Check sheet for the drawn part. Datum: minimum x, y, z corner. Units: mm. Coordinates: 2 decimals unless noted, no trailing zeros. Loops run counter-clockwise (first coordinate to the right, second up) from the corner with the lowest first, then second, coordinate; pieces in that order, holes last.
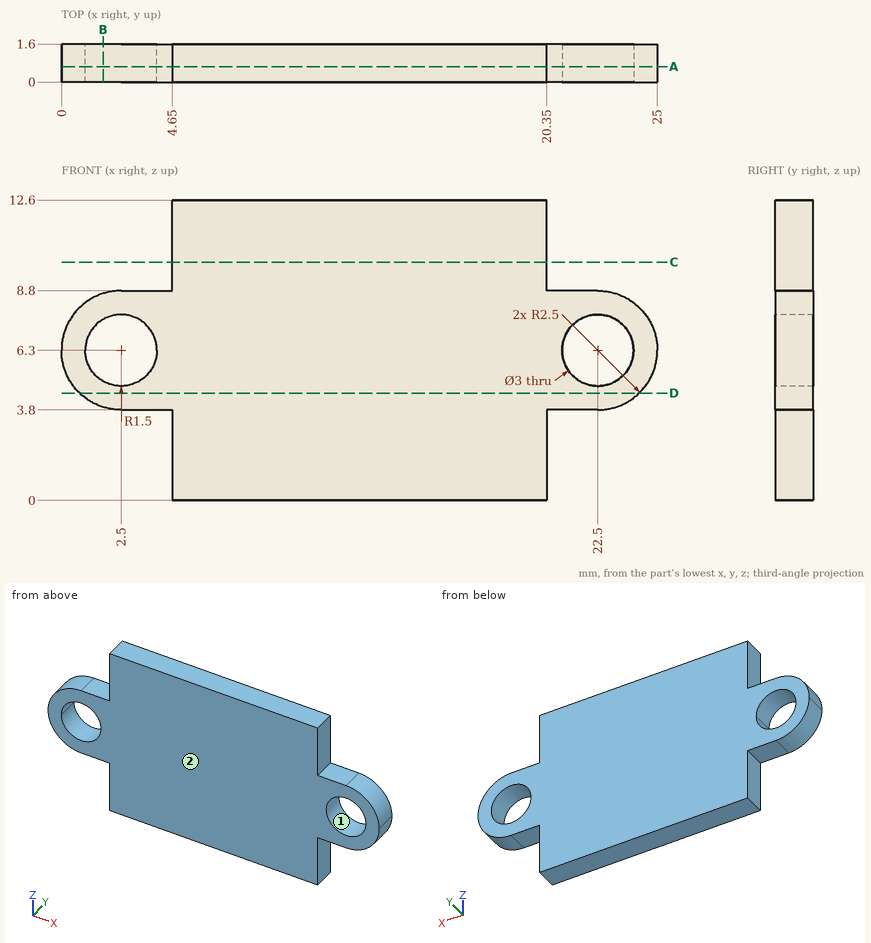
1) Section check C-C on z = 10. Enter the section's corners in (x, y), plus the area to 3 significant figures.
Answer sheet:
outline: (4.65, 0) - (20.35, 0) - (20.35, 1.6) - (4.65, 1.6) - close
area: 25.1 mm2
2) Mould release check, pull along X, two halves, no side actions. Record for the marked faces 1 and 2: +X half, -X half, draft (parallel to the pull), parting line (faces both ways), or undercut.
Answer sheet:
face 1: undercut
face 2: draft
3) Section check B-B on x = 1.75. Enter the section's corners in (y, z).
Answer sheet:
outline: (0, 3.92) - (1.6, 3.92) - (1.6, 5) - (0, 5) - close; (0, 7.6) - (1.6, 7.6) - (1.6, 8.68) - (0, 8.68) - close
4) Section check D-D on z = 4.5. Enter the section's corners in (x, y).
Answer sheet:
outline: (0.77, 0) - (24.23, 0) - (24.23, 1.6) - (0.77, 1.6) - close
5) Section check A-A on y = 0.65. Enter the section's corners in (x, z).
Answer sheet:
outline: (2.5, 3.8) - (4.65, 3.8) - (4.65, 0) - (20.35, 0) - (20.35, 3.8) - (22.5, 3.8) arc R2.5 ccw to (22.5, 8.8) - (20.35, 8.8) - (20.35, 12.6) - (4.65, 12.6) - (4.65, 8.8) - (2.5, 8.8) arc R2.5 ccw to start; hole circle Ø3 at (2.5, 6.3); hole circle Ø3 at (22.5, 6.3)
6) Depth check by flat-ended pin: pin 1 (0.5 mm diameter, centred on x = 21, y = 0.5, fed in from +Z); pin 2 (0.5 mm diameter, centred on x = 3.5, y = 1, fed in from -Z); pin 3 (0.8 mm diameter, centred on y = 1, z = 10.5, fed in from +X); pin 4 (1.8 mm diameter, centred on x = 22.5, z = 6.3, fed in from -Y). Enter the tip coordinate at first touch or a pass-through.
Answer sheet:
pin 1: stops at z = 8.8
pin 2: stops at z = 3.8
pin 3: stops at x = 20.35
pin 4: passes through
7) Scan lines: line 1 (X direction, y = 1.1, z = 6.3); line 2 (X direction, y = 1, z = 5); line 3 (X direction, y = 1.55, z = 11). Record each from-to range of solid material in increasing order.
Answer sheet:
line 1: x = 0 to 1, 4 to 21, 24 to 25
line 2: x = 0.36 to 1.75, 3.25 to 21.75, 23.25 to 24.64
line 3: x = 4.65 to 20.35
